Check sheet for the modelled part. Datum: model origin and axes. Units: mm. Face numbers are marked on the shaded views. A direction names the side the tool comes from. Coordinates: 2 decimals unless noted, no trailing zeros. Write each loop counter-clockwise with the first axis right and the second up, starting at its lowest first coordinate (ties: lowest second). Pieces come first, ordered by that corner, then holes. Notation, with made-up numbers: (38.25, -40) -> (43.25, -40) arc R10 ccw to (43.25, -21) -> close; hole circle Ø5 at (55.5, 54). An arc over 180 degrees is marked (long way). One line per item, written item: value. Start each with the question number.
1) Gauge pin test, flat end, axial feed: P1, Ø3, axis at y = 1.5, z = -36, coming from the +X side. Record the tip position at first contact, or that the pin passes through.
2) Scan lines: line 1 along Z through (x, y) = (-1.5, 0); line 2 along Z through (x, y) = (-2.25, 0.25); line 3 along Z through (x, y) = (-1.5, 2.5). Record each from-to range of solid material in increasing order. Write a range as [from, to].
3) Sectioned sample at C-C on x = 0.5. Enter the section's corners in (y, z).
4) Sectioned sample at D-D on z = -31. Enter the section's corners in (x, y).
5) Sectioned sample at B-B on y = 0. Enter the section's corners in (x, z).
6) Set-up check for the marked faces 1 and 2: record each of +Z, -Z, +X, -X, +Y, -Y from which the full face is reachable in a straight line by a thin tool's end or side.
7) Sectioned sample at A-A on x = 2.5. Enter the section's corners in (y, z).
```python
from build123d import *

# Parameters (mm, degrees)
SKETCH_2_R               = 1.5
CUT_EXTRUDE_1_DEPTH      = 4
CUT_EXTRUDE_1_DEPTH_BACK = 4


with BuildPart() as part:
    # 草圖1 → 旋轉1 (revolve)
    with BuildSketch(Plane(origin=(0, 0, 0), x_dir=(0, 0, -1), z_dir=(1, 0, 0))):
        Polygon((0, 2), (0, 3), (-13, 3), (-13, 0), (43, 0), (43, 3), (40, 3), (40, 2), align=None)
    revolve(axis=Axis((0, 0, 17.804347826), (0, 0, -1)))

    # 草圖2 → 除料-伸長1 (cut, two sides)
    with BuildSketch(Plane(origin=(0, 0, 0), x_dir=(0, 0, -1), z_dir=(1, 0, 0))) as cut_extrude_1_sk:
        with Locations((-10, 0)):
            Circle(SKETCH_2_R)
    extrude(amount=CUT_EXTRUDE_1_DEPTH, mode=Mode.SUBTRACT)
    extrude(cut_extrude_1_sk.sketch, amount=-CUT_EXTRUDE_1_DEPTH_BACK, mode=Mode.SUBTRACT)


solid = part.part
```
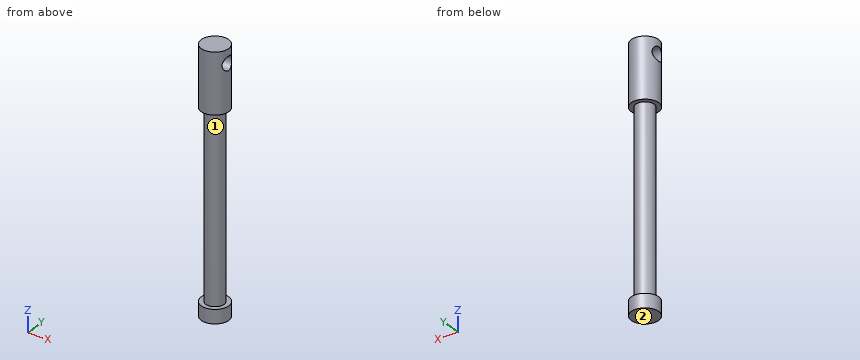
Answers:
1. P1: stops at x = 2
2. line 1: z = [-43, 8.5], [11.5, 13]
2. line 2: z = [-43, -40], [0, 8.52], [11.48, 13]
2. line 3: z = [-43, -40], [0, 13]
3. outline: (-2.96, -43) -> (2.96, -43) -> (2.96, -40) -> (1.94, -40) -> (1.94, 0) -> (2.96, 0) -> (2.96, 13) -> (-2.96, 13) -> (-2.96, 0) -> (-1.94, 0) -> (-1.94, -40) -> (-2.96, -40) -> close; hole circle Ø3 at (0, 10)
4. outline: circle Ø4 at (0, 0)
5. outline: (-3, -43) -> (3, -43) -> (3, -40) -> (2, -40) -> (2, 0) -> (3, 0) -> (3, 8.5) -> (-3, 8.5) -> (-3, 0) -> (-2, 0) -> (-2, -40) -> (-3, -40) -> close; (-3, 11.5) -> (3, 11.5) -> (3, 13) -> (-3, 13) -> close
6. face 1: none
6. face 2: -Z, +X, -X, +Y, -Y
7. outline: (-1.66, -43) -> (1.66, -43) -> (1.66, -40) -> (-1.66, -40) -> close; (-1.66, 0) -> (1.66, 0) -> (1.66, 13) -> (-1.66, 13) -> close; hole circle Ø3 at (0, 10)
